```python
from build123d import *

# Parameters (mm, degrees)
BOSS_EXTRUDE1_DEPTH = 5.08
SKETCH3_W           = 4.826
SKETCH3_H           = 6.35076331
SKETCH3_W_2         = 6.35
SKETCH3_H_2         = 5.08
CUT_EXTRUDE1_DEPTH  = 6.0800001


with BuildPart() as part:
    # Sketch2 → Boss-Extrude1 (new body)
    with BuildSketch(Plane.XY):
        with BuildLine():
            Line((158.75, -0.200025), (158.75, 0.200025))
            add(Edge.make_bspline(
                [(158.75, 0.200025), (156.104769639, 0.564899501), (150.817056987, 1.294269442), (142.878358215, 2.306719234), (134.940769513, 3.268408227), (127.002836924, 4.172206586), (119.065195908, 5.02492376), (111.127662782, 5.825402282), (103.190287717, 6.571495389), (95.252619427, 7.253962327), (87.315238521, 7.873917198), (79.324754405, 8.420599463), (71.334509538, 8.88842609), (63.343416227, 9.23480821), (55.458296632, 9.48903948), (50.217735657, 9.487192482), (47.625, 9.52576331)],
                knots=[0, 0, 0, 0, 0.024634231, 0.04924287, 0.07382978, 0.098396751, 0.122945996, 0.147478562, 0.171994581, 0.196493552, 0.220976186, 0.245442093, 0.270380478, 0.294812969, 0.319231823, 0.343153728, 0.343153728, 0.343153728, 0.343153728], degree=3))
            Line((47.625, 9.52576331), (47.625, -9.52576331))
            add(Edge.make_bspline(
                [(47.625, -9.52576331), (50.217735657, -9.487192482), (55.458296632, -9.48903948), (63.343416227, -9.23480821), (71.334509538, -8.88842609), (79.324754405, -8.420599463), (87.315238521, -7.873917198), (95.252619427, -7.253962327), (103.190287717, -6.571495389), (111.127662782, -5.825402282), (119.065195908, -5.02492376), (127.002836924, -4.172206586), (134.940769513, -3.268408227), (142.878358215, -2.306719234), (150.817056987, -1.294269442), (156.104769639, -0.564899501), (158.75, -0.200025)],
                knots=[0.656846272, 0.656846272, 0.656846272, 0.656846272, 0.680768177, 0.705187031, 0.729619522, 0.754557907, 0.779023814, 0.803506448, 0.828005419, 0.852521438, 0.877054004, 0.901603249, 0.92617022, 0.95075713, 0.975365769, 1, 1, 1, 1], degree=3))
        make_face()
    extrude(amount=BOSS_EXTRUDE1_DEPTH)

    # Sketch3 → Cut-Extrude1 (cut, through all)
    with BuildSketch(Plane(origin=(0, 0, 0), x_dir=(-1, 0, 0), z_dir=(0, 0, -1))):
        with Locations((-50.038, -6.350381655)):
            Rectangle(SKETCH3_W, SKETCH3_H)
        with Locations((-50.038, 6.350381655)):
            Rectangle(SKETCH3_W, SKETCH3_H)
        with Locations((-68.326, 0)):
            Rectangle(SKETCH3_W_2, SKETCH3_H_2)
    extrude(amount=-CUT_EXTRUDE1_DEPTH, mode=Mode.SUBTRACT)


solid = part.part
```
Verification items for the finished model (mm, model axes). A direction names the side the tool comes from. Coordinates: 2 decimals unless noted, no trailing zeros. Put each result on its own line as item: value.
1. Thickness scan on line 1 (Y direction, x = 149, z = 0.45); line 2 (Y direction, x = 107.5, z = 4.2). Record the ranges inside material, lowest first.
Result set:
line 1: y = -1.52 to 1.52
line 2: y = -6.16 to 6.16
2. Tool access check on faces 1 (the face through (90, 0, 5.08)), 2 (the face through (52.451, -6, 3)), 3 (the face through (50, 3.175, 3)), 4 (the face through (65.151, 0, 3)). Record the directions out of +Z, -Z, +X, -X, +Y, -Y that give a thin tool (end or side, any length) a straight path to the whole face; none if there is none.
Result set:
face 1: +Z, +X, -X, +Y, -Y
face 2: +Z, -Z, -X, -Y
face 3: +Z, -Z, -X, +Y
face 4: +Z, -Z
3. Gauge pin test, flat ends, axial feed: P1, Ø2, axis at x = 102.5, z = 4, coming from the -Y side; P2, Ø1.4, axis at x = 50.5, z = 3.5, coming from the +Y side (3 decimals); P3, Ø1.4, axis at x = 50.5, z = 2.5, coming from the -Y side (3 decimals). Record the tip position at first contact, or that the pin passes through.
Result set:
P1: stops at y = -6.71
P2: stops at y = 3.175
P3: stops at y = -3.175
4. Mould release check, pull along X, two halves, no side actions. Record for faces 5 (the face through (68, -2.54, 3)), 6 (the face through (90, 0, 0)), 7 (the face through (47.625, 0, 3)), 8 (the face through (71.501, 0, 3)): pulls with the +X half, pulls with the -X half, needs draft (parallel to the pull), parting line crosses it, or undercut.
Result set:
face 5: undercut
face 6: needs draft
face 7: pulls with the -X half
face 8: undercut
